Geometry check sheet. Reference: drawing and pictorial views, mm from the part's lowest x, y, z. Coordinates: 2 decimals unless noted, no trailing zeros. Loops run counter-clockwise (first coordinate to the right, second up) from the corner with the lowest first, then second, coordinate; pieces in that order, holes last. Notation, with made-up numbers: M -0.75,22 L 48.25,22 A7 ccw 48.25,33 Z; hole C 67,20.5 d4. An arc over 180 degrees is marked long. Write each question's results on one line, items separated by ' | '. Start each with the question number.
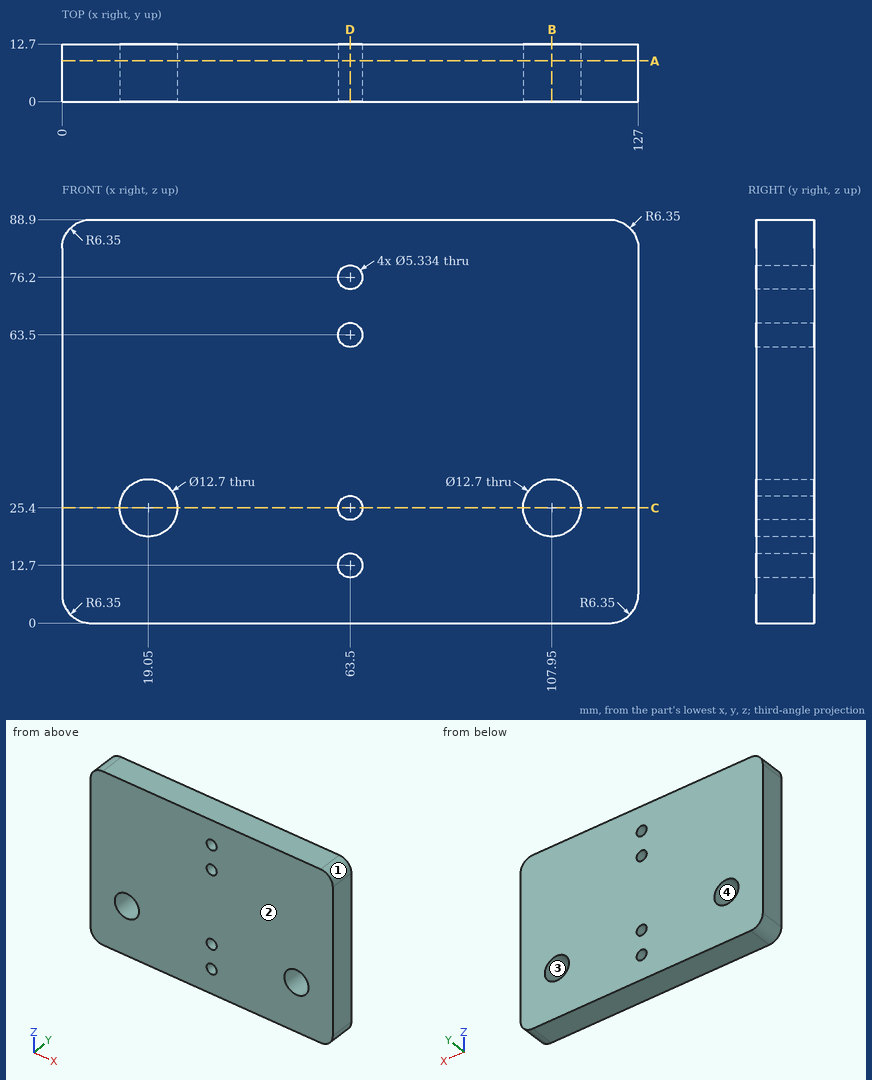
1) Section check B-B (x = 107.95). Enter the section's corners in (y, z), then the cut area to 3 significant figures.
2) Section check A-A (y = 9). Enter the section's corners in (x, z), then the cut area to 3 significant figures.
3) Section check C-C (z = 25.4). Enter the section's corners in (x, y).
4) Gauge pin test, flat end, axial feed: P1, Ø5, axis at x = 63.5, z = 12.7, coming from the -Y side. Record the tip position at first contact, or that the pin passes through.
5) Section check D-D (x = 63.5). Enter the section's corners in (y, z), then the cut area to 3 significant figures.
6) Release check for a two-part mould opening along Z. For the marked faces 1, 2, 3 and 4 record: +Z half, -Z half, draft (parallel to the pull), parting line (faces both ways), or undercut.
7) Thickness scan on probe 1 along X at (y, z) = (3.75, 25.4); probe 2 along X at (y, z) = (6.25, 12.7); probe 3 along Z at (x, y) = (21, 1.75). Record the ranges inside material, lowest first.
Return value:
1) outline: M 0,0 L 12.7,0 L 12.7,19.05 L 0,19.05 Z; M 0,31.75 L 12.7,31.75 L 12.7,88.9 L 0,88.9 Z | area: 968 mm2
2) outline: M 0,6.35 A6.35 ccw 6.35,0 L 120.65,0 A6.35 ccw 127,6.35 L 127,82.55 A6.35 ccw 120.65,88.9 L 6.35,88.9 A6.35 ccw 0,82.55 Z; hole C 19.05,25.4 d12.7; hole C 63.5,12.7 d5.33; hole C 63.5,25.4 d5.33; hole C 63.5,63.5 d5.33; hole C 63.5,76.2 d5.33; hole C 107.95,25.4 d12.7 | area: 10,900 mm2
3) outline: M 0,0 L 12.7,0 L 12.7,12.7 L 0,12.7 Z; M 25.4,0 L 60.83,0 L 60.83,12.7 L 25.4,12.7 Z; M 66.17,0 L 101.6,0 L 101.6,12.7 L 66.17,12.7 Z; M 114.3,0 L 127,0 L 127,12.7 L 114.3,12.7 Z
4) P1: passes through
5) outline: M 0,0 L 12.7,0 L 12.7,10.03 L 0,10.03 Z; M 0,15.37 L 12.7,15.37 L 12.7,22.73 L 0,22.73 Z; M 0,28.07 L 12.7,28.07 L 12.7,60.83 L 0,60.83 Z; M 0,66.17 L 12.7,66.17 L 12.7,73.53 L 0,73.53 Z; M 0,78.87 L 12.7,78.87 L 12.7,88.9 L 0,88.9 Z | area: 858 mm2
6) face 1: +Z half | face 2: draft | face 3: undercut | face 4: undercut
7) probe 1: x = 0 to 12.7, 25.4 to 60.83, 66.17 to 101.6, 114.3 to 127 | probe 2: x = 0 to 60.83, 66.17 to 127 | probe 3: z = 0 to 19.36, 31.44 to 88.9
